from build123d import *

# Parameters (mm, degrees)
F0_W      = 44
F0_H      = 44
F1_DEPTH  = 25
F0_W_2    = 264
F0_H_2    = 264
F4_DEPTH  = 50
F3_FACE_W = 44
F3_FACE_H = 25
F1_FACE_W = 44
F1_FACE_H = 25
F2_FACE_W = 44
F2_FACE_H = 25
F5_DEPTH  = 44
F6_DEPTH  = 22


with BuildPart() as f1:
    # F0 (on Top) → F1 (new body)
    with BuildSketch(Plane.XY):
        with Locations((-88, 0)):
            Rectangle(F0_W, F0_H)
    extrude(amount=F1_DEPTH)


with BuildPart() as f1b:
    # F0 (on Top) → F1, piece 2 (new body)
    with BuildSketch(Plane.XY):
        with Locations((-88, 88)):
            Rectangle(F0_W, F0_H)
    extrude(amount=F1_DEPTH)


with BuildPart() as f1c:
    # F0 (on Top) → F1, piece 3 (new body)
    with BuildSketch(Plane.XY):
        with Locations((0, 88)):
            Rectangle(F0_W, F0_H)
    extrude(amount=F1_DEPTH)


with BuildPart() as f1d:
    # F0 (on Top) → F1, piece 4 (new body)
    with BuildSketch(Plane.XY):
        Rectangle(F0_W, F0_H)
    extrude(amount=F1_DEPTH)


with BuildPart() as f2_1:
    # F2: instance of F1
    add(f1.part.mirror(Plane.YZ))


with BuildPart() as f2_2:
    # F2: instance of F1b
    add(f1b.part.mirror(Plane.YZ))


with BuildPart() as f3_1:
    # F3: instance of F1b
    add(f1b.part.mirror(Plane.XZ))


with BuildPart() as f3_2:
    # F3: instance of F1c
    add(f1c.part.mirror(Plane.XZ))


with BuildPart() as f3_3:
    # F3: instance of F2_2
    add(f2_2.part.mirror(Plane.XZ))


with BuildPart() as f4:
    # F0 (on Top) → F4 (new body)
    with BuildSketch(Plane.XY):
        Rectangle(F0_W_2, F0_H_2)
        with Locations((-88, 0)):
            Rectangle(F0_W, F0_H, mode=Mode.SUBTRACT)
        with Locations((-88, 88)):
            Rectangle(F0_W, F0_H, mode=Mode.SUBTRACT)
        Rectangle(F0_W, F0_H, mode=Mode.SUBTRACT)
        with Locations((0, 88)):
            Rectangle(F0_W, F0_H, mode=Mode.SUBTRACT)
        with Locations((-88, 0)):
            Rectangle(F0_W, F0_H)
        Rectangle(F0_W, F0_H)
        with Locations((-88, 88)):
            Rectangle(F0_W, F0_H)
        with Locations((0, 88)):
            Rectangle(F0_W, F0_H)
    extrude(amount=-F4_DEPTH)


with BuildPart() as f1_1:
    add(f1.part)

    add(f1b.part)  # F5 merges F1b

    add(f1c.part)  # F5 merges F1c

    add(f1d.part)  # F5 merges F1d

    add(f2_1.part)  # F5 merges F2_1

    add(f2_2.part)  # F5 merges F2_2

    add(f3_1.part)  # F5 merges F3_1

    add(f3_2.part)  # F5 merges F3_2

    add(f3_3.part)  # F5 merges F3_3

    add(f4.part)  # F5 merges F4
    # F3_face (on face) + F1_face (on face) + F2_face (on face) → F5 (join)
    with BuildSketch(Plane(origin=(-88, -66, 12.5), x_dir=(-1, 0, 0), z_dir=(0, 1, 0))):
        Rectangle(F3_FACE_W, F3_FACE_H)
        with Locations((-88, 0)):
            Rectangle(F3_FACE_W, F3_FACE_H)
        with Locations((-176, 0)):
            Rectangle(F3_FACE_W, F3_FACE_H)
    with BuildSketch(Plane(origin=(-88, 22, 12.5), x_dir=(-1, 0, 0), z_dir=(0, 1, 0))):
        Rectangle(F1_FACE_W, F1_FACE_H)
        with Locations((-88, 0)):
            Rectangle(F1_FACE_W, F1_FACE_H)
    with BuildSketch(Plane(origin=(88, 22, 12.5), x_dir=(-1, 0, 0), z_dir=(0, 1, 0))):
        Rectangle(F2_FACE_W, F2_FACE_H)
    extrude(amount=F5_DEPTH)

    # F6 (add, symmetric): faces of the model
    f6_faces = [f1_1.faces().sort_by_distance(p)[0] for p in [
        (-88, -110, 12.5),
        (0, -110, 12.5),
        (88, -110, 12.5),
        (-88, 110, 12.5),
        (0, 110, 12.5),
        (88, 110, 12.5),
    ]]
    extrude(f6_faces, amount=F6_DEPTH, both=True, dir=(0, -1, 0))


solid = f1_1.part
Part model, mm, in its own coordinate system. A direction names the side the tool comes from. Round coordinates to 2 decimals unless told otherwise and drop trailing zeros. Write each loop counter-clockwise with the first axis right and the second up, starting at its lowest first coordinate (ties: lowest second). Pieces come first, ordered by that corner, then holes. Notation, with made-up numbers: M 75.5,-11.5 L 133.5,-11.5 A21 cw 133.5,15.5 Z; hole C 75,68 d11. An arc over 180 degrees is marked long. Return JSON: item names as keys, results as strings. Group by question number.
(1) Drill centre lines: probe 1 along X at (y, z) = (42, 8); probe 2 along Z at (x, y) = (118, 107). Where is each one in solid material? Low to high.
(2) Saw through at C-C on x = 31.5. Write the cut outline in (y, z), then the cut area to 3 significant figures.
(3) Saw through at A-A on z = 20.5. Write the cut outline in (x, y).
(4) Two-plate mould, pull along X, no slides. Class faces 1 (the face through (-44, 2, 0)), 2 (the face through (-132, -2, -25)), 3 (the face through (66, -2, 12)), 4 (the face through (110, -2, 12)): +X half, -X half, draft (parallel to the pull), parting line (faces both ways), or undercut.
(5) Which spindle directions (+Z, -Z, +X, -X, +Y, -Y) get a long thin tool onto all of the face, cutting with end or side? Do faces 5 (the face through (-110, 2, 12)), 6 (the face through (121, 2, 0)), 7 (the face through (-22, 2, 12)). Say none if no direction does.
(6) Saw through at B-B on y = 39.5. Write the cut outline in (x, z).
(7) Pin check, flat tips, straight feed: pin 1 Ø13 at (x, y) = (-43.5, 12) entering from +Z; pin 2 Ø12.5 at (y, z) = (-18, 7.5) entering from +X; pin 3 Ø7.5 at (y, z) = (43, 13.5) entering from -X; pin 4 Ø20 at (y, z) = (0, 7.5) entering from +X. Stop position of each tip, or through.
Returned:
{
 "1": {"probe 1": "-110 to -66, -22 to 22, 66 to 110", "probe 2": "-50 to 0"},
 "2": {"outline": "M -132,-50 L 132,-50 L 132,0 L -132,0 Z", "area": "13,200 mm²"},
 "3": {"outline": "M -110,-132 L -66,-132 L -66,132 L -110,132 Z; M -22,-132 L 22,-132 L 22,132 L -22,132 Z; M 66,-132 L 110,-132 L 110,132 L 66,132 Z"},
 "4": {"face 1": "undercut", "face 2": "-X half", "face 3": "undercut", "face 4": "+X half"},
 "5": {"face 5": "+Z, -X, +Y, -Y", "face 6": "+Z, +X, +Y, -Y", "face 7": "+Z, +Y, -Y"},
 "6": {"outline": "M -132,-50 L 132,-50 L 132,0 L 110,0 L 110,25 L 66,25 L 66,0 L 22,0 L 22,25 L -22,25 L -22,0 L -66,0 L -66,25 L -110,25 L -110,0 L -132,0 Z"},
 "7": {"pin 1": "z = 0", "pin 2": "x = 110", "pin 3": "x = -110", "pin 4": "x = 132"}
}
